Input: part model. Units: mm. Frame: model coordinates. Face numbers are marked on the shaded views. A direction names the side the tool comes from. Round coordinates to 2 decimals unless told otherwise and drop trailing zeros. Order: outer loops, then holes, each group sorted by start corner. A loop starts at its lowest first (then second) coordinate and runs counter-clockwise, first axis right, second up. Notation, with made-up numbers: (-34, 1.5) -> (9, 1.5) arc R9 cw to (9, 9.5) -> close; hole circle Ø3 at (52, -23). An arc over 180 degrees is marked (long way). Use a Markdown table: item, result.
from build123d import *

# Parameters (mm, degrees)
SKETCH1_W           = 29.21
SKETCH1_H           = 21.59
BOSS_EXTRUDE1_DEPTH = 101.6
SKETCH2_W           = 44.45
SKETCH2_H           = 21.59
SKETCH2_R           = 1.5875
BOSS_EXTRUDE2_DEPTH = 6.35
FILLET1_R           = 1.27
SKETCH3_W           = 11.43
SKETCH3_H           = 190.5
CUT_EXTRUDE1_DEPTH  = 113.3088653
FILLET2_R           = 3.81


with BuildPart() as part:
    # Sketch1 → Boss-Extrude1 (new, symmetric)
    with BuildSketch(Plane.XY):
        Rectangle(SKETCH1_W, SKETCH1_H)
    extrude(amount=BOSS_EXTRUDE1_DEPTH, both=True)

    # Sketch2 → Boss-Extrude2 (add)
    with BuildSketch(Plane.XY.offset(101.6)):
        Rectangle(SKETCH2_W, SKETCH2_H)
        with Locations((-19.05, 6.35)):
            Circle(SKETCH2_R, mode=Mode.SUBTRACT)
        with Locations(Location((-19.05, -6.35, 0), (0, 0, 180))):
            Circle(SKETCH2_R, mode=Mode.SUBTRACT)
        with Locations((19.05, -6.35)):
            Circle(SKETCH2_R, mode=Mode.SUBTRACT)
        with Locations(Location((19.05, 6.35, 0), (0, 0, 180))):
            Circle(SKETCH2_R, mode=Mode.SUBTRACT)
    boss_extrude2 = extrude(amount=BOSS_EXTRUDE2_DEPTH)

    # Mirror1: Boss-Extrude2 across plane
    add(boss_extrude2.mirror(Plane.XY))

    # Fillet1
    fillet1_edges = [part.edges().sort_by_distance(p)[0] for p in [
        (14.605, 0, 101.6),
        (-14.605, 0, 101.6),
        (14.605, 0, -101.6),
        (-14.605, 0, -101.6),
    ]]
    fillet(fillet1_edges, radius=FILLET1_R)

    # Sketch3 → Cut-Extrude1 (cut, through all)
    with BuildSketch(Plane(origin=(0, 10.795, 0), x_dir=(1, 0, 0), z_dir=(0, 1, 0))):
        Rectangle(SKETCH3_W, SKETCH3_H)
    extrude(amount=-CUT_EXTRUDE1_DEPTH, mode=Mode.SUBTRACT)

    # Fillet2
    fillet2_edges = [part.edges().sort_by_distance(p)[0] for p in [
        (-5.715, 0, -95.25),
        (5.715, 0, -95.25),
        (5.715, 0, 95.25),
        (-5.715, 0, 95.25),
    ]]
    fillet(fillet2_edges, radius=FILLET2_R)


solid = part.part
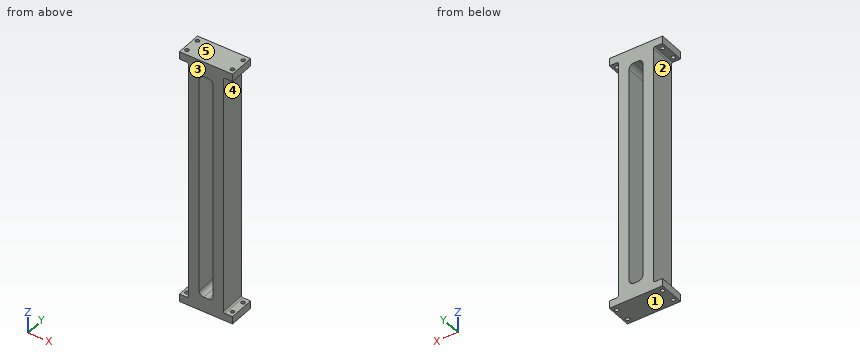
1) Draft query along Z for the marked faces 1, 2 and 3. Return one class per face: released by +Z, released by -Z, zero draft, split by the parting line, or undercut.
Answer key:
| item | result |
|---|---|
| face 1 | released by -Z |
| face 2 | undercut |
| face 3 | zero draft |
2) Ray query, probe 1 along Y at (x, z) = (19, 104) (3 decimals); probe 2 along X at (y, z) = (-4, 3) (3 decimals); probe 3 along Z at (x, y) = (2, -7). Return the intervals inside material, ascending.
Answer key:
| item | result |
|---|---|
| probe 1 | y = -10.795 to -7.937, -4.763 to 4.763, 7.937 to 10.795 |
| probe 2 | x = -14.605 to -5.715, 5.715 to 14.605 |
| probe 3 | z = -107.95 to -95.25, 95.25 to 107.95 |
3) Cut plane B-B on z = 41.5. Return loops of the section in (x, y) (3 decimals), and give its area (3 significant figures).
Answer key:
| item | result |
|---|---|
| outline | (-14.605, -10.795) -> (-5.715, -10.795) -> (-5.715, 10.795) -> (-14.605, 10.795) -> close; (5.715, -10.795) -> (14.605, -10.795) -> (14.605, 10.795) -> (5.715, 10.795) -> close |
| area | 384 mm^2 |
4) Contact query for flat-ended pins moving along their axis: P1, Ø5, axis at y = -2, z = -14, coming from the -X side (3 decimals); P2, Ø4, axis at y = -5, z = -31.5, coming from the +X side (3 decimals); P3, Ø5, axis at x = -19.05, y = 6.35, coming from the +Z side. Output: stop coordinate, or through.
Answer key:
| item | result |
|---|---|
| P1 | stops at x = -14.605 |
| P2 | stops at x = 14.605 |
| P3 | stops at z = 107.95 |
5) Cut plane A-A on y = 0. Return loops of the section in (x, z) (3 decimals).
Answer key:
| item | result |
|---|---|
| outline | (-22.225, -107.95) -> (22.225, -107.95) -> (22.225, -101.6) -> (15.875, -101.6) arc R1.27 cw to (14.605, -100.33) -> (14.605, 100.33) arc R1.27 cw to (15.875, 101.6) -> (22.225, 101.6) -> (22.225, 107.95) -> (-22.225, 107.95) -> (-22.225, 101.6) -> (-15.875, 101.6) arc R1.27 cw to (-14.605, 100.33) -> (-14.605, -100.33) arc R1.27 cw to (-15.875, -101.6) -> (-22.225, -101.6) -> close; hole (-5.715, -91.44) arc R3.81 ccw to (-1.905, -95.25) -> (1.905, -95.25) arc R3.81 ccw to (5.715, -91.44) -> (5.715, 91.44) arc R3.81 ccw to (1.905, 95.25) -> (-1.905, 95.25) arc R3.81 ccw to (-5.715, 91.44) -> close |
6) Set-up query: the marked faces 4 and 5. Return all of +Z, -Z, +X, -X, +Y, -Y with unobstructed straight access to the full face (end or side cutting, diameter ignored); none if empty.
Answer key:
| item | result |
|---|---|
| face 4 | +X, +Y, -Y |
| face 5 | +Z, +X, -X, +Y, -Y |
